Could you check a few things on this model? Use its own coordinates, in mm. A direction names the side the tool comes from. Coordinates: 2 decimals unless noted, no trailing zeros. Write each loop counter-clockwise with the first axis right and the second up, starting at its lowest first coordinate (ties: lowest second). Pieces come first, ordered by that corner, then holes.
Item 1: I want a section at A-A on x = 0. Please give me the cut outline in (y, z).
Item 2: Which directions (+Z, -Z, +X, -X, +Y, -Y) give clear straight access to the entire face, cutting with the end or side of a thin tool? Please do faces 1 (the flat face through (0, -8, 10)), 2 (the flat face through (2.1, 2.4, 12)).
Item 3: If I drill on probe 1 along Y at (x, z) = (0, 3.75); probe 2 along Z at (x, y) = (-1.25, -8.25); probe 3 along Y at (x, z) = (2.25, 1.5), over which ranges is the centre line in solid material (lowest first)?
Item 4: I want a section at C-C on z = 5.25. Please give me the cut outline in (x, y), then the cut area to 3 significant figures.
Item 5: Thinking about a two-plate mould opening in Y: for faces 3 (the flat face through (2.5, -2.5, 0)), 4 (the cylindrical face through (3, 0, 6)), 5 (the cylindrical face through (-1.009, 7.684, 5.944)), which applies, +Y half, -Y half, draft (parallel to the pull), parting line (faces both ways), or undercut?
Item 6: I want a section at D-D on y = 8. Please give me the cut outline in (x, z).
Item 7: For P1, Ø1, axis at y = -5.5, z = 6, coming from the -X side; P2, Ø1, axis at x = 7, z = 8, coming from the -Y side; P3, Ø1.5, axis at x = -6.5, z = 4, coming from the -Y side, each with a flat end and sliding along its axis, tell me the tip position at first contact or that it passes through.
from build123d import *

# Parameters (mm, degrees)
SKETCH1_R           = 7.75
SKETCH1_R_2         = 2.5
BOSS_EXTRUDE1_DEPTH = 12
SKETCH2_R           = 9.95
SKETCH2_R_2         = 3
BOSS_EXTRUDE2_DEPTH = 2
CHAMFER1_SIZE       = 2
SKETCH3_R           = 3
CUT_EXTRUDE1_DEPTH  = 13


with BuildPart() as part:
    # Sketch1 → Boss-Extrude1 (new body)
    with BuildSketch(Plane.XY):
        Circle(SKETCH1_R)
        Circle(SKETCH1_R_2, mode=Mode.SUBTRACT)
    extrude(amount=BOSS_EXTRUDE1_DEPTH)

    # Sketch2 → Boss-Extrude2 (add)
    with BuildSketch(Plane.XY.offset(12)):
        Circle(SKETCH2_R)
        Circle(SKETCH2_R_2, mode=Mode.SUBTRACT)
    extrude(amount=-BOSS_EXTRUDE2_DEPTH)

    # Chamfer1
    chamfer1_edges = [part.edges().sort_by_distance(p)[0] for p in [
        (-7.75, 0, 0),
    ]]
    chamfer(chamfer1_edges, length=CHAMFER1_SIZE)

    # Sketch3 → Cut-Extrude1 (cut, through all)
    with BuildSketch(Plane(origin=(0, 0, 0), x_dir=(-1, 0, 0), z_dir=(0, 0, -1))):
        Circle(SKETCH3_R)
    extrude(amount=-CUT_EXTRUDE1_DEPTH, mode=Mode.SUBTRACT)


solid = part.part
Response values:
1. outline: (-9.95, 10) - (-7.75, 10) - (-7.75, 2) - (-5.75, 0) - (-3, 0) - (-3, 12) - (-9.95, 12) - close; (3, 0) - (5.75, 0) - (7.75, 2) - (7.75, 10) - (9.95, 10) - (9.95, 12) - (3, 12) - close
2. face 1: -Z
2. face 2: +Z, +X, -X, +Y, -Y
3. probe 1: y = -7.75 to -3, 3 to 7.75
3. probe 2: z = 10 to 12
3. probe 3: y = -6.89 to -1.98, 1.98 to 6.89
4. outline: circle Ø15.5 at (0, 0); hole circle Ø6 at (0, 0)
4. area: 160 mm2
5. face 3: draft
5. face 4: undercut
5. face 5: parting line
6. outline: (-5.92, 10) - (5.92, 10) - (5.92, 12) - (-5.92, 12) - close
7. P1: stops at x = -5.92
7. P2: stops at y = -4.22
7. P3: stops at y = -5.2
